Design review of the part built by this model. Coordinates are the model's own, in mm. Face numbers are marked on the shaded views. A direction names the side the tool comes from. Coordinates: 2 decimals unless noted, no trailing zeros. Write each loop counter-clockwise with the first axis right and the second up, starting at its lowest first coordinate (ties: lowest second). Pieces come first, ordered by that corner, then holes.
Q1. Insertion check: pin 1 (5 mm diameter, centred on x = -21, z = 1, fed in from +Y); pin 2 (1 mm diameter, centred on x = -4, y = 91.5, fed in from -Z); pin 3 (6 mm diameter, centred on x = -46, y = 82.5, fed in from +Z). Each pin has a flat end and moves straight along its axis. Give the tip position at first contact, or say it passes through.
Q2. Take a section at A-A (z = 13). Give the boundary of the cut face in (x, y).
Q3. Take a section at C-C (y = 7.5). Give the boundary of the cut face in (x, z), and give its area (3 significant figures).
Q4. Take a section at D-D (z = 53). Give the boundary of the cut face in (x, y) (3 decimals), and give its area (3 significant figures).
Q5. Machinability: for the marked faces 1, 2, 3, 4 and 5, which of the approach directions +Z, -Z, +X, -X, +Y, -Y give a long, thin tool a straight path to every point of the face, cutting with its end or side? Answer none if there is none.
Q6. Mouldability with a two-part tool opening along X and no side actions: class the marked faces 6, 7, 8 and 9 as pulls with the +X half, pulls with the -X half, needs draft (parallel to the pull), parting line crosses it, or undercut.
Q7. Take a section at B-B (x = 5). Give the boundary of the cut face in (y, z) (3 decimals), and give its area (3 significant figures).
Q8. For probe 1 along Y at (x, z) = (-45.5, 28.5); probe 2 along Y at (x, z) = (-25.5, 45.5) (3 decimals); probe 3 along X at (y, z) = (19, 48), list the stretches that pass through material, from the lowest coordinate up.
Autodesk Inventor part; units mm, degrees
ref_plane "YZ Plane" through (0, 0, 0) normal (1, 0, 0) x (0, 1, 0)
ref_plane "XZ Plane" through (0, 0, 0) normal (0, 1, 0) x (-1, 0, 0)
ref_plane "XY Plane" through (0, 0, 0) normal (0, 0, 1) x (1, 0, 0)
sketch "Sketch1" plane through (0, 0, 0) normal (0, 1, 0) x (-1, 0, 0)
  line L0 (48.2977, 71.5211) -> (-16.7023, 71.5211)
  line L1 (-16.7023, 71.5211) -> (-16.7023, -8.4789)
  line L2 (-16.7023, -8.4789) -> (48.2977, -8.4789)
  line L3 (48.2977, -8.4789) -> (48.2977, 71.5211)
  arc A0 (22.2975, -8.4789) -> (-2.7023, -8.4789) centre (9.7976, -8.4281) ccw
  line L4 (-16.7023, -8.4789) -> (-11.7023, -8.4789)
  line L5 (-11.7023, -8.4789) -> (-11.7023, 71.5211)
  line L6 (-11.7023, 71.5211) -> (-16.7023, 71.5211)
  line L7 (-16.7023, 71.5211) -> (-16.7023, -8.4789)
  line L8 (48.2977, -8.4789) -> (40.7977, -8.4789)
  line L9 (40.7977, -8.4789) -> (40.7977, 71.5211)
  line L10 (40.7977, 71.5211) -> (48.2977, 71.5211)
  line L11 (48.2977, 71.5211) -> (48.2977, -8.4789)
  line L12 (-11.7023, -8.4789) -> (40.7977, -8.4789)
  line L13 (40.7977, -8.4789) -> (40.7977, 9.0211)
  line L14 (40.7977, 9.0211) -> (-11.7023, 9.0211)
  line L15 (-11.7023, 9.0211) -> (-11.7023, -8.4789)
  line L16 (-11.7023, 71.5211) -> (40.7977, 71.5211)
  line L17 (40.7977, 71.5211) -> (40.7977, 64.0211)
  line L18 (40.7977, 64.0211) -> (-11.7023, 64.0211)
  line L19 (-11.7023, 64.0211) -> (-11.7023, 71.5211)
  line L20 (-16.7023, 61.5211) -> (-6.7023, 71.5211)
  line L21 (-16.7023, 61.5211) -> (-16.7023, 71.5211)
  line L22 (-6.7023, 71.5211) -> (-11.7023, 66.5211)
  line L23 (-11.7023, 64.0211) -> (-11.7023, 66.5211)
  line L24 (-6.7023, 71.5211) -> (40.7977, 71.5211)
  line L25 (40.7977, 64.0211) -> (-11.7023, 64.0211)
  line L26 (-11.7023, 66.5211) -> (-11.7023, 64.0211)
  line L27 (-11.7023, 66.5211) -> (-6.7023, 71.5211)
  line L28 (-11.7023, 54.0211) -> (-1.7023, 64.0211)
  point P0 (0, 0)
  dimension "d0" = 80
  dimension "d1" = 65
  dimension "d3" = 14
  dimension "d4" = 12.5
  dimension "d5" = 7.5
  dimension "d6" = 5
  dimension "d7" = 17.5
  dimension "d8" = 7.5
  dimension "d9" = 10
  dimension "d10" = 10
  dimension "d48" = 10
  dimension "d49" = 10
extrude "Extrusion1" add sketch "Sketch1" along normal blind 110 contours L3 L2 L9 L0 | L9 L18 L5 L20 L0 | L2 A0 L5 L14 L9 | L5 L2 L1 L20
sketch "Sketch2" plane through (-22.2975, 0, -8.4789) normal (0, 0, -1) x (-1, 0, 0)
  line L0 (18.5002, 0) -> (18.5002, 110)
  line L1 (18.5002, 110) -> (-33.9998, 110)
  line L2 (-33.9998, 110) -> (-33.9998, 10)
  line L3 (-33.9998, 10) -> (18.5002, 10)
  line L4 (18.5002, 10) -> (18.5002, 110)
  point P0 (-22.2975, 0)
  dimension "d13" = 100
  dimension "d14" = 52.5
extrude "Extrusion2" cut sketch "Sketch2" against normal blind 30
sketch "Sketch3" plane through (-40.7977, 0, 9.0211) normal (0, 0, 1) x (1, 0, 0)
  line L0 (52.5, 10) -> (0, 10)
  line L1 (26.0002, 10) -> (36, 10)
  line L2 (18.5002, 10) -> (18.5002, 0)
  line L3 (43.5, 0) -> (43.5, 10)
  line L4 (0, 0) -> (52.5, 0)
  line L5 (38.5, 0) -> (23.5002, 0)
  line L6 (23.5002, 0) -> (23.5002, 5)
  line L7 (23.5002, 5) -> (38.5, 5)
  line L8 (38.5, 5) -> (38.5, 0)
  point P0 (40.7977, 0)
  dimension "d43" = 5
  dimension "d44" = 5
  dimension "d45" = 5
sketch "Sketch4" plane through (16.7023, 0, 61.5211) normal (1, 0, 0) x (0, 0, -1)
  line L0 (70, 110) -> (70, 10)
  line L1 (70, 94) -> (36, 94)
  line L2 (36, 94) -> (36, 16)
  line L3 (36, 16) -> (70, 16)
  line L4 (70, 16) -> (70, 94)
  line L5 (0, 0) -> (70, 0)
  line L6 (0, 110) -> (70, 110)
  point P0 (61.5211, 0)
  dimension "d22" = 34
  dimension "d23" = 16
  dimension "d24" = 16
  dimension "d25" = 78
extrude "Extrusion4" cut sketch "Sketch4" against normal blind 30
sketch "Sketch5" plane through (0, 0, 0) normal (0, -1, 0) x (1, 0, 0)
  line L0 (-40.7977, -8.4789) -> (-22.2975, -8.4789)
  arc A0 (-40.2975, -8.4789) -> (-37.2975, -8.4789) centre (-38.7975, -8.4789) ccw
  arc A1 (-37.2975, -8.4789) -> (-40.2975, -8.4789) centre (-38.7975, -8.4789) ccw
  point P0 (0, 0)
  dimension "d28" = 18
  dimension "d29" = 1.5
  dimension "d30" = 0
  dimension "d31" = 1.5
extrude "Extrusion5" cut sketch "Sketch5" against normal blind 30 contours A1 L0
sketch "Sketch7" plane through (-48.2977, 0, 71.5211) normal (0, 0, 1) x (1, 0, 0)
  line L0 (0, 110) -> (55, 110)
  line L1 (0, 110) -> (40, 110)
  line L2 (40, 110) -> (0, 60)
  line L3 (0, 60) -> (0, 110)
  line L4 (65, 110) -> (65, 0)
  point P0 (48.2977, 0)
  dimension "d39" = 40
  dimension "d40" = 25
  dimension "d41" = 50
extrude "Extrusion6" cut sketch "Sketch3" against normal blind 30 contours L4 L6 L7 L8
sketch "Sketch8" plane through (0, 110, 0) normal (0, 1, 0) x (1, 0, 0)
  line L0 (11.7023, 8.4789) -> (11.7023, -64.0211)
  line L1 (11.7023, -59.0211) -> (6.7023, -64.0211)
  line L2 (6.7023, -64.0211) -> (11.7023, -64.0211)
  line L3 (11.7023, -64.0211) -> (11.7023, -59.0211)
  point P0 (0, 0)
  dimension "d50" = 5
  dimension "d51" = 5
extrude "Extrusion7" add sketch "Sketch8" against normal up to surface (110 mm away)
extrude "Extrusion8" cut sketch "Sketch7" against normal blind 30
sketch "Sketch9" plane through (11.7023, 0, 9.0211) normal (-1, 0, 0) x (0, 0, 1)
  line L0 (32.5, 69.375) -> (55, 69.375)
  line L1 (50, 0) -> (50, 110)
  line L2 (50, 69.375) -> (25, 69.375)
  line L3 (25, 69.375) -> (25, 54.375)
  line L4 (25, 54.375) -> (50, 54.375)
  line L5 (50, 54.375) -> (50, 69.375)
  point P0 (-9.0211, 0)
  dimension "d56" = 15
  dimension "d57" = 25
sketch "Sketch11" plane through (11.7023, 0, 9.0211) normal (-1, 0, 0) x (0, 0, 1)
  line L0 (-17.5, 94) -> (-17.5, 110)
  line L1 (-17.5, 100) -> (12.5, 100)
  line L2 (12.5, 100) -> (12.5, 103.5)
  line L3 (12.5, 103.5) -> (-17.5, 103.5)
  line L4 (-17.5, 103.5) -> (-17.5, 100)
  line L5 (-17.5, 110) -> (50, 110)
  point P0 (-9.0211, 0)
  dimension "d62" = 3.5
  dimension "d63" = 30
  dimension "d64" = 10
extrude "Extrusion11" add sketch "Sketch11" along normal up to next
sketch "Sketch12" plane through (-48.2977, 0, -8.4789) normal (-1, 0, 0) x (0, 0, 1)
  line L0 (0, 100) -> (0, 10)
  line L1 (0, 52.5) -> (60, 52.5)
  line L2 (60, 52.5) -> (60, 25)
  line L3 (60, 25) -> (0, 25)
  line L4 (0, 25) -> (0, 52.5)
  line L5 (80, 0) -> (80, 60)
  line L6 (80, 60) -> (50, 60)
  point P0 (8.4789, 0)
  dimension "d67" = 27.5
  dimension "d68" = 60
  dimension "d69" = 20
  dimension "d70" = 7.5
extrude "Extrusion12" cut sketch "Sketch12" against normal up to surface (60 mm away)
sketch "Sketch13" plane through (11.7023, 0, 9.0211) normal (-1, 0, 0) x (0, 0, 1)
  line L0 (0, 0) -> (50, 0)
  line L1 (50, 0) -> (32.154, 0)
  line L2 (32.154, 0) -> (32.154, 10.7503)
  line L3 (32.154, 10.7503) -> (50, 10.7503)
  line L4 (50, 10.7503) -> (50, 0)
  point P0 (-9.0211, 0)
sketch "Sketch14" plane through (6.7023, 0, 64.0211) normal (0, 0, -1) x (-1, 0, 0)
  point P0 (6.7023, 0)
extrude "Extrusion13" add sketch "Sketch9" along normal up to next
extrude "Extrusion14" add sketch "Sketch13" along normal up to next
sketch "Sketch15" plane through (-40.7977, 0, 59.0211) normal (0, 0, 1) x (1, 0, 0)
  line L0 (0, 0) -> (0, 10.7503)
  line L1 (52.5, 0) -> (0, 0)
  line L2 (52.5, 0) -> (52.5, 10.7503)
  line L3 (52.5, 10.7503) -> (0, 10.7503)
  line L4 (52.5, 0) -> (52.5, 10.7503)
  line L5 (52.5, 0) -> (0, 0)
  line L6 (0, 54.375) -> (0, 69.375)
  line L7 (52.5, 54.375) -> (0, 54.375)
  line L8 (52.5, 54.375) -> (52.5, 69.375)
  line L9 (52.5, 69.375) -> (0, 69.375)
  point P0 (40.7977, 0)
extrude "Extrusion15" add sketch "Sketch15" along normal blind 5.5
equation "\"d8\" = d5"
equation "\"d49\" = d48"
equation "\"d44\" = d43"
equation "\"d24\" = d23"
equation "\"d31\" = d29"
equation "\"d50\" = d51"
properties part number "Basev3.3"
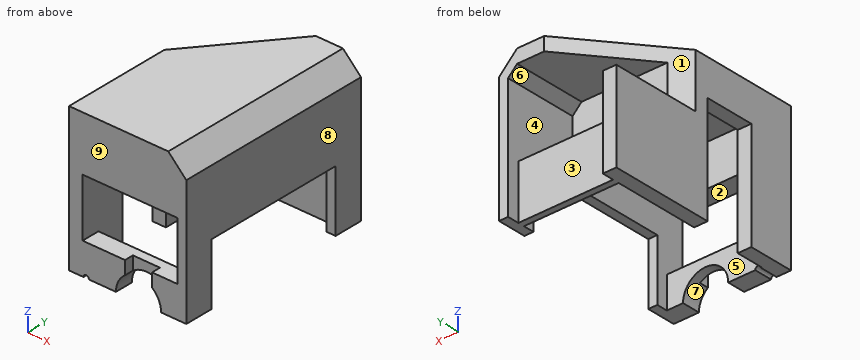
Response:
1. pin 1: stops at y = 103.5
1. pin 2: stops at z = 64.02
1. pin 3: stops at z = 41.52
2. outline: (-48.3, 0) - (-40.8, 0) - (-40.8, 25) - (-48.3, 25) - close; (-48.3, 52.5) - (-40.8, 52.5) - (-40.8, 100) - (11.7, 100) - (11.7, 94) - (16.7, 94) - (16.7, 110) - (11.7, 110) - (11.7, 103.5) - (-40.8, 103.5) - (-40.8, 110) - (-48.3, 110) - close; (11.7, 0) - (16.7, 0) - (16.7, 16) - (11.7, 16) - close
3. outline: (-48.3, -8.48) - (-40.3, -8.48) arc R1.5 cw to (-37.3, -8.48) - (-22.3, -8.48) arc R12.5 cw (long way) to (2.7, -8.48) - (16.7, -8.48) - (16.7, 61.52) - (6.7, 71.52) - (-48.3, 71.52) - close; hole (-40.8, 9.02) - (11.7, 9.02) - (11.7, 41.18) - (-40.8, 41.18) - close
3. area: 3,210 mm2
4. outline: (-48.298, 0) - (16.702, 0) - (16.702, 110) - (11.702, 110) - (11.702, 69.375) - (-40.798, 69.375) - (-48.298, 60) - close; hole (-40.798, 10.75) - (11.702, 10.75) - (11.702, 54.375) - (-40.798, 54.375) - close
4. area: 2,390 mm2
5. face 1: +Z, -X, +Y
5. face 2: -Y
5. face 3: -Z, +Y
5. face 4: none
5. face 5: -Z
6. face 6: pulls with the -X half
6. face 7: undercut
6. face 8: pulls with the +X half
6. face 9: needs draft
7. outline: (0, -8.479) - (10, -8.479) - (10, 9.021) - (0, 9.021) - close; (0, 41.175) - (10.75, 41.175) - (10.75, 64.021) - (54.375, 64.021) - (54.375, 34.021) - (69.375, 34.021) - (69.375, 64.021) - (110, 64.021) - (110, 71.521) - (0, 71.521) - close; (100, -8.479) - (103.5, -8.479) - (103.5, 21.521) - (100, 21.521) - close
7. area: 1,800 mm2
8. probe 1: y = 0 to 25, 52.5 to 110
8. probe 2: y = 0 to 10.75, 54.375 to 69.375
8. probe 3: x = -48.3 to -40.8, 11.7 to 16.7
